Part model, mm, in its own coordinate system. Round coordinates to 2 decimals unless told otherwise and drop trailing zeros. Loops run counter-clockwise (first coordinate to the right, second up) from the corner with the lowest first, then second, coordinate; pieces in that order, holes last.
(1) Cut at C-C on x = 469.5. List the corners of the cut face in (y, z).
(2) Cut at A-A on x = 457. List the corners of the cut face in (y, z).
(3) Cut at B-B on x = 419. List the corners of the cut face in (y, z).
(4) Cut at D-D on y = 43. List the corners of the cut face in (x, z).
(5) Probe probe 1 along Y at (x, z) = (416.5, -0.9); probe 2 along Y at (x, z) = (468.5, 0.3); probe 3 along X at (y, z) = (70.5, 0.55). List the from-to ranges inside material, lowest first.
from build123d import *

# Parameters (mm, degrees)
SALIENTE_EXTRUIR1_START = -1.5
SALIENTE_EXTRUIR1_DEPTH = 3
CROQUIS4_W              = 23.371648172
CROQUIS4_H              = 47.52448784
CORTAR_EXTRUIR3_DEPTH   = 10
CROQUIS5_W              = 9.999999994
CROQUIS5_H              = 3
CROQUIS5_W_2            = 9.999999993
CORTAR_EXTRUIR4_DEPTH   = 10
CROQUIS6_R              = 1.5
CROQUIS6_R_2            = 3.5
CORTAR_EXTRUIR5_DEPTH   = 10
REDONDEO1_R             = 5


# Read off the part's stored shape, not the designer's step: Saliente-Extruir1
with BuildPart() as part:
    # Saliente-Extruir1 outline → Saliente-Extruir1 (new body)
    with BuildSketch(Plane.XY.offset(SALIENTE_EXTRUIR1_START)):
        with BuildLine():
            ThreePointArc((492.916449572, 98.009593947), (492.452410006, 99.442022929), (491.249851225, 100.348134338))
            ThreePointArc((491.249851225, 100.348134338), (487.916517891, 105.062179546), (491.249851225, 109.776224754))
            ThreePointArc((491.249851225, 109.776224754), (492.452037009, 110.681812922), (492.916439741, 112.113480025))
            Line((492.916439741, 112.113480025), (492.916413331, 149.999679341))
            Line((492.916413331, 149.999679341), (410.416517891, 149.999679341))
            Line((410.416517891, 149.999679341), (410.416517891, 112.133247358))
            ThreePointArc((410.416517891, 112.133247358), (410.875276439, 110.689871685), (412.083184558, 109.776224754))
            ThreePointArc((412.083184558, 109.776224754), (415.416517891, 105.062179546), (412.083184558, 100.348134338))
            ThreePointArc((412.083184558, 100.348134338), (410.875276439, 99.434487407), (410.416517891, 97.991111734))
            Line((410.416517891, 97.991111734), (410.416517891, 52.008362374))
            ThreePointArc((410.416517891, 52.008362374), (410.875276439, 50.564986701), (412.083184558, 49.65133977))
            ThreePointArc((412.083184558, 49.65133977), (415.416517891, 44.937294562), (412.083184558, 40.223249354))
            ThreePointArc((412.083184558, 40.223249354), (410.875276439, 39.309602423), (410.416517891, 37.86622675))
            Line((410.416517891, 37.86622675), (410.416517891, -0.000320659))
            Line((410.416517891, -0.000320659), (492.916517891, -0.000320659))
            Line((492.916517891, -0.000320659), (492.916491488, 37.877716604))
            ThreePointArc((492.916491488, 37.877716604), (492.45443711, 39.314289338), (491.249851225, 40.223249354))
            ThreePointArc((491.249851225, 40.223249354), (487.916517891, 44.937294562), (491.249851225, 49.65133977))
            ThreePointArc((491.249851225, 49.65133977), (492.453865854, 50.559496169), (492.916481647, 51.994900607))
            Line((492.916481647, 51.994900607), (492.916449572, 98.009593947))
        make_face()
    extrude(amount=SALIENTE_EXTRUIR1_DEPTH)

    # Croquis4 → Cortar-Extruir3 (cut)
    with BuildSketch(Plane.XY.offset(1.5)):
        with Locations((455.222459901, 75.336681949)):
            Rectangle(CROQUIS4_W, CROQUIS4_H)
    extrude(amount=-CORTAR_EXTRUIR3_DEPTH, mode=Mode.SUBTRACT)

    # Croquis5 → Cortar-Extruir4 (cut)
    with BuildSketch(Plane(origin=(0, 0, -1.5), x_dir=(-1, 0, 0), z_dir=(0, 0, -1))):
        with Locations((-420.416517885, 27.399679341)):
            Rectangle(CROQUIS5_W, CROQUIS5_H)
        with Locations((-480.50829052, 27.399679341)):
            Rectangle(CROQUIS5_W_2, CROQUIS5_H)
        with Locations((-480.50829052, 122.599679342)):
            Rectangle(CROQUIS5_W_2, CROQUIS5_H)
        with Locations((-420.416517885, 122.599679342)):
            Rectangle(CROQUIS5_W, CROQUIS5_H)
    extrude(amount=-CORTAR_EXTRUIR4_DEPTH, mode=Mode.SUBTRACT)

    # Croquis6 → Cortar-Extruir5 (cut)
    with BuildSketch(Plane.XY.offset(1.5)):
        with Locations((460.461664074, 27.503843939)):
            Circle(CROQUIS6_R)
        with Locations((440.404261852, 27.568711017)):
            Circle(CROQUIS6_R)
        with Locations((468.41649135, 38.074679341)):
            Circle(CROQUIS6_R_2)
        with Locations((468.416510711, 10.299679341)):
            Circle(CROQUIS6_R_2)
        with Locations((440.404261852, 122.435783537)):
            Circle(CROQUIS6_R)
        with Locations((460.461664074, 122.500650615)):
            Circle(CROQUIS6_R)
        with Locations((468.41649135, 133.074679341)):
            Circle(CROQUIS6_R_2)
        with Locations((468.416510711, 105.299679341)):
            Circle(CROQUIS6_R_2)
    extrude(amount=-CORTAR_EXTRUIR5_DEPTH, mode=Mode.SUBTRACT)

    # Redondeo1
    redondeo1_edges = [part.edges().sort_by_distance(p)[0] for p in [
        (466.908283987, 99.098925869, 0),
        (466.908283987, 51.574438029, 0),
        (443.536635815, 51.574438029, 0),
        (443.536635815, 99.098925869, 0),
    ]]
    fillet(redondeo1_edges, radius=REDONDEO1_R)


solid = part.part
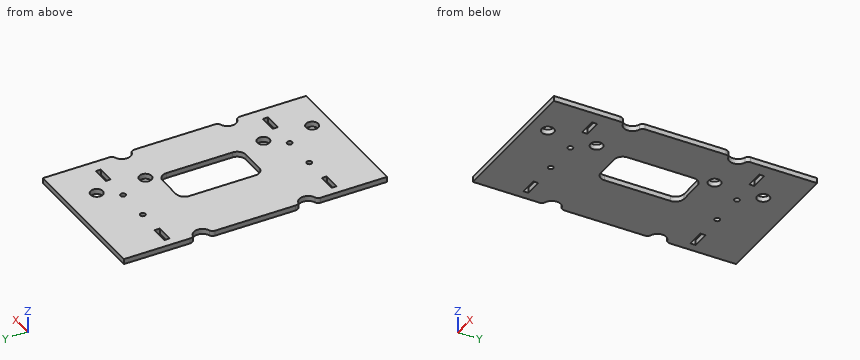
Final values:
1. outline: (0, -1.5) - (6.97, -1.5) - (6.97, 1.5) - (0, 1.5) - close; (13.63, -1.5) - (34.75, -1.5) - (34.75, 1.5) - (13.63, 1.5) - close; (41.4, -1.5) - (101.97, -1.5) - (101.97, 1.5) - (41.4, 1.5) - close; (108.63, -1.5) - (129.75, -1.5) - (129.75, 1.5) - (108.63, 1.5) - close; (136.4, -1.5) - (150, -1.5) - (150, 1.5) - (136.4, 1.5) - close
2. outline: (0, -1.5) - (51.57, -1.5) - (51.57, 1.5) - (0, 1.5) - close; (99.1, -1.5) - (150, -1.5) - (150, 1.5) - (99.1, 1.5) - close
3. outline: (0, -1.5) - (25.9, -1.5) - (25.9, 1.5) - (0, 1.5) - close; (28.9, -1.5) - (121.1, -1.5) - (121.1, 1.5) - (28.9, 1.5) - close; (124.1, -1.5) - (150, -1.5) - (150, 1.5) - (124.1, 1.5) - close
4. outline: (415.03, -1.5) - (488.31, -1.5) - (488.31, 1.5) - (415.03, 1.5) - close
5. probe 1: y = 0 to 25.9, 28.9 to 121.1, 124.1 to 150
5. probe 2: y = 0 to 6.8, 13.8 to 34.58, 41.57 to 101.8, 108.8 to 129.58, 136.57 to 150
5. probe 3: x = 410.42 to 443.54, 466.91 to 492.92
